```python
from build123d import *

# Parameters (mm, degrees)
F0_W             = 25.4
F0_H             = 25.4
F1_DEPTH         = 12.7
F3_D             = 3.175
F5_D             = 3.175
F7_D             = 3.175
F11_D            = 17.145
F11_DEPTH        = 3.81
F11_TIP          = 5.1508776566
F11_ON_F6_D      = 17.145
F11_ON_F6_DEPTH  = 3.81
F11_ON_F6_TIP    = 5.1508776566
F11_ON_F10_D     = 17.145
F11_ON_F10_DEPTH = 3.81
F11_ON_F10_TIP   = 5.1508776566
F11_ON_F4_D      = 17.145
F11_ON_F4_DEPTH  = 3.81
F11_ON_F4_TIP    = 5.1508776566
F11_ON_F9_D      = 17.145
F11_ON_F9_DEPTH  = 3.81
F11_ON_F9_TIP    = 5.1508776566
F11_ON_F2_D      = 17.145
F11_ON_F2_DEPTH  = 3.81
F11_ON_F2_TIP    = 5.1508776566
F12_D            = 22.225
F12_DEPTH        = 0.635
F12_TIP          = 6.6770636289
F12_ON_F2_D      = 22.225
F12_ON_F2_DEPTH  = 0.635
F12_ON_F2_TIP    = 6.6770636289
F12_ON_F10_D     = 22.225
F12_ON_F10_DEPTH = 0.635
F12_ON_F10_TIP   = 6.6770636289
F12_ON_F8_D      = 22.225
F12_ON_F8_DEPTH  = 0.635
F12_ON_F8_TIP    = 6.6770636289
F12_ON_F4_D      = 22.225
F12_ON_F4_DEPTH  = 0.635
F12_ON_F4_TIP    = 6.6770636289
F12_ON_F6_D      = 22.225
F12_ON_F6_DEPTH  = 0.635
F12_ON_F6_TIP    = 6.6770636289
F13_D            = 12.065
F13_DEPTH        = 3.81
F13_START        = 5.336186
F13_TIP          = 3.6246916843
F13_ON_F8_D      = 12.065
F13_ON_F8_DEPTH  = 3.81
F13_ON_F8_START  = 5.336186
F13_ON_F8_TIP    = 3.6246916843
F13_ON_F10_D     = 12.065
F13_ON_F10_DEPTH = 3.81
F13_ON_F10_START = 5.336186
F13_ON_F10_TIP   = 3.6246916843
F13_ON_F9_D      = 12.065
F13_ON_F9_DEPTH  = 3.81
F13_ON_F9_START  = 5.336186
F13_ON_F9_TIP    = 3.6246916843
F13_ON_F6_D      = 12.065
F13_ON_F6_DEPTH  = 3.81
F13_ON_F6_START  = 5.336186
F13_ON_F6_TIP    = 3.6246916843
F13_ON_F2_D      = 12.065
F13_ON_F2_DEPTH  = 3.81
F13_ON_F2_START  = 5.336186
F13_ON_F2_TIP    = 3.6246916843


with BuildPart() as f1:
    # F0 (on Top) → F1 (new body, symmetric)
    with BuildSketch(Plane.XY):
        Rectangle(F0_W, F0_H)
    extrude(amount=F1_DEPTH, both=True)

    # F3 (through all)
    with Locations(Plane.XY.offset(12.7)):
        with Locations((0, 0)):
            Hole(F3_D / 2)

    # F5 (through all)
    with Locations(Plane(origin=(-12.7, 0, 0), x_dir=(0, -1, 0), z_dir=(-1, 0, 0))):
        with Locations((0, 0)):
            Hole(F5_D / 2)

    # F7 (through all)
    with Locations(Plane(origin=(0, 12.7, 0), x_dir=(-1, 0, 0), z_dir=(0, 1, 0))):
        with Locations((0, 0)):
            Hole(F7_D / 2)

    # F11
    with Locations(Plane(origin=(0, 0, -12.7), x_dir=(1, 0, 0), z_dir=(0, 0, -1))):
        with Locations((0, 0)):
            Hole(F11_D / 2, depth=F11_DEPTH)
            with Locations((0, 0, -(F11_DEPTH + F11_TIP / 2))):  # 118° drill point
                Cone(0, F11_D / 2, F11_TIP, mode=Mode.SUBTRACT)

    # F11 on F6
    with Locations(Plane(origin=(0, 12.7, 0), x_dir=(-1, 0, 0), z_dir=(0, 1, 0))):
        with Locations((0, 0)):
            Hole(F11_ON_F6_D / 2, depth=F11_ON_F6_DEPTH)
            with Locations((0, 0, -(F11_ON_F6_DEPTH + F11_ON_F6_TIP / 2))):  # 118° drill point
                Cone(0, F11_ON_F6_D / 2, F11_ON_F6_TIP, mode=Mode.SUBTRACT)

    # F11 on F10
    with Locations(Plane.XZ.offset(12.7)):
        with Locations((0, 0)):
            Hole(F11_ON_F10_D / 2, depth=F11_ON_F10_DEPTH)
            with Locations((0, 0, -(F11_ON_F10_DEPTH + F11_ON_F10_TIP / 2))):  # 118° drill point
                Cone(0, F11_ON_F10_D / 2, F11_ON_F10_TIP, mode=Mode.SUBTRACT)

    # F11 on F4
    with Locations(Plane(origin=(-12.7, 0, 0), x_dir=(0, -1, 0), z_dir=(-1, 0, 0))):
        with Locations((0, 0)):
            Hole(F11_ON_F4_D / 2, depth=F11_ON_F4_DEPTH)
            with Locations((0, 0, -(F11_ON_F4_DEPTH + F11_ON_F4_TIP / 2))):  # 118° drill point
                Cone(0, F11_ON_F4_D / 2, F11_ON_F4_TIP, mode=Mode.SUBTRACT)

    # F11 on F9
    with Locations(Plane.YZ.offset(12.7)):
        with Locations((0, 0)):
            Hole(F11_ON_F9_D / 2, depth=F11_ON_F9_DEPTH)
            with Locations((0, 0, -(F11_ON_F9_DEPTH + F11_ON_F9_TIP / 2))):  # 118° drill point
                Cone(0, F11_ON_F9_D / 2, F11_ON_F9_TIP, mode=Mode.SUBTRACT)

    # F11 on F2
    with Locations(Plane.XY.offset(12.7)):
        with Locations((0, 0)):
            Hole(F11_ON_F2_D / 2, depth=F11_ON_F2_DEPTH)
            with Locations((0, 0, -(F11_ON_F2_DEPTH + F11_ON_F2_TIP / 2))):  # 118° drill point
                Cone(0, F11_ON_F2_D / 2, F11_ON_F2_TIP, mode=Mode.SUBTRACT)

    # F12
    with Locations(Plane.YZ.offset(12.7)):
        with Locations((0, 0)):
            Hole(F12_D / 2, depth=F12_DEPTH)
            with Locations((0, 0, -(F12_DEPTH + F12_TIP / 2))):  # 118° drill point
                Cone(0, F12_D / 2, F12_TIP, mode=Mode.SUBTRACT)

    # F12 on F2
    with Locations(Plane.XY.offset(12.7)):
        with Locations((0, 0)):
            Hole(F12_ON_F2_D / 2, depth=F12_ON_F2_DEPTH)
            with Locations((0, 0, -(F12_ON_F2_DEPTH + F12_ON_F2_TIP / 2))):  # 118° drill point
                Cone(0, F12_ON_F2_D / 2, F12_ON_F2_TIP, mode=Mode.SUBTRACT)

    # F12 on F10
    with Locations(Plane.XZ.offset(12.7)):
        with Locations((0, 0)):
            Hole(F12_ON_F10_D / 2, depth=F12_ON_F10_DEPTH)
            with Locations((0, 0, -(F12_ON_F10_DEPTH + F12_ON_F10_TIP / 2))):  # 118° drill point
                Cone(0, F12_ON_F10_D / 2, F12_ON_F10_TIP, mode=Mode.SUBTRACT)

    # F12 on F8
    with Locations(Plane(origin=(0, 0, -12.7), x_dir=(1, 0, 0), z_dir=(0, 0, -1))):
        with Locations((0, 0)):
            Hole(F12_ON_F8_D / 2, depth=F12_ON_F8_DEPTH)
            with Locations((0, 0, -(F12_ON_F8_DEPTH + F12_ON_F8_TIP / 2))):  # 118° drill point
                Cone(0, F12_ON_F8_D / 2, F12_ON_F8_TIP, mode=Mode.SUBTRACT)

    # F12 on F4
    with Locations(Plane(origin=(-12.7, 0, 0), x_dir=(0, -1, 0), z_dir=(-1, 0, 0))):
        with Locations((0, 0)):
            Hole(F12_ON_F4_D / 2, depth=F12_ON_F4_DEPTH)
            with Locations((0, 0, -(F12_ON_F4_DEPTH + F12_ON_F4_TIP / 2))):  # 118° drill point
                Cone(0, F12_ON_F4_D / 2, F12_ON_F4_TIP, mode=Mode.SUBTRACT)

    # F12 on F6
    with Locations(Plane(origin=(0, 12.7, 0), x_dir=(-1, 0, 0), z_dir=(0, 1, 0))):
        with Locations((0, 0)):
            Hole(F12_ON_F6_D / 2, depth=F12_ON_F6_DEPTH)
            with Locations((0, 0, -(F12_ON_F6_DEPTH + F12_ON_F6_TIP / 2))):  # 118° drill point
                Cone(0, F12_ON_F6_D / 2, F12_ON_F6_TIP, mode=Mode.SUBTRACT)

    # F13
    # its depths count from where the whole tool has entered the part; down to there all is cleared
    with Locations(Plane(origin=(-12.7, 0, 0), x_dir=(0, -1, 0), z_dir=(-1, 0, 0))):
        with Locations((0, 0)):
            Hole(F13_D / 2, depth=F13_START)
    with Locations(Plane(origin=(-12.7, 0, 0), x_dir=(0, -1, 0), z_dir=(-1, 0, 0)).offset(-F13_START)):
        with Locations((0, 0)):
            Hole(F13_D / 2, depth=F13_DEPTH)
            with Locations((0, 0, -(F13_DEPTH + F13_TIP / 2))):  # 118° drill point
                Cone(0, F13_D / 2, F13_TIP, mode=Mode.SUBTRACT)

    # F13 on F8
    # its depths count from where the whole tool has entered the part; down to there all is cleared
    with Locations(Plane(origin=(0, 0, -12.7), x_dir=(1, 0, 0), z_dir=(0, 0, -1))):
        with Locations((0, 0)):
            Hole(F13_ON_F8_D / 2, depth=F13_ON_F8_START)
    with Locations(Plane(origin=(0, 0, -12.7), x_dir=(1, 0, 0), z_dir=(0, 0, -1)).offset(-F13_ON_F8_START)):
        with Locations((0, 0)):
            Hole(F13_ON_F8_D / 2, depth=F13_ON_F8_DEPTH)
            with Locations((0, 0, -(F13_ON_F8_DEPTH + F13_ON_F8_TIP / 2))):  # 118° drill point
                Cone(0, F13_ON_F8_D / 2, F13_ON_F8_TIP, mode=Mode.SUBTRACT)

    # F13 on F10
    # its depths count from where the whole tool has entered the part; down to there all is cleared
    with Locations(Plane.XZ.offset(12.7)):
        with Locations((0, 0)):
            Hole(F13_ON_F10_D / 2, depth=F13_ON_F10_START)
    with Locations(Plane.XZ.offset(12.7).offset(-F13_ON_F10_START)):
        with Locations((0, 0)):
            Hole(F13_ON_F10_D / 2, depth=F13_ON_F10_DEPTH)
            with Locations((0, 0, -(F13_ON_F10_DEPTH + F13_ON_F10_TIP / 2))):  # 118° drill point
                Cone(0, F13_ON_F10_D / 2, F13_ON_F10_TIP, mode=Mode.SUBTRACT)

    # F13 on F9
    # its depths count from where the whole tool has entered the part; down to there all is cleared
    with Locations(Plane.YZ.offset(12.7)):
        with Locations((0, 0)):
            Hole(F13_ON_F9_D / 2, depth=F13_ON_F9_START)
    with Locations(Plane.YZ.offset(12.7).offset(-F13_ON_F9_START)):
        with Locations((0, 0)):
            Hole(F13_ON_F9_D / 2, depth=F13_ON_F9_DEPTH)
            with Locations((0, 0, -(F13_ON_F9_DEPTH + F13_ON_F9_TIP / 2))):  # 118° drill point
                Cone(0, F13_ON_F9_D / 2, F13_ON_F9_TIP, mode=Mode.SUBTRACT)

    # F13 on F6
    # its depths count from where the whole tool has entered the part; down to there all is cleared
    with Locations(Plane(origin=(0, 12.7, 0), x_dir=(-1, 0, 0), z_dir=(0, 1, 0))):
        with Locations((0, 0)):
            Hole(F13_ON_F6_D / 2, depth=F13_ON_F6_START)
    with Locations(Plane(origin=(0, 12.7, 0), x_dir=(-1, 0, 0), z_dir=(0, 1, 0)).offset(-F13_ON_F6_START)):
        with Locations((0, 0)):
            Hole(F13_ON_F6_D / 2, depth=F13_ON_F6_DEPTH)
            with Locations((0, 0, -(F13_ON_F6_DEPTH + F13_ON_F6_TIP / 2))):  # 118° drill point
                Cone(0, F13_ON_F6_D / 2, F13_ON_F6_TIP, mode=Mode.SUBTRACT)

    # F13 on F2
    # its depths count from where the whole tool has entered the part; down to there all is cleared
    with Locations(Plane.XY.offset(12.7)):
        with Locations((0, 0)):
            Hole(F13_ON_F2_D / 2, depth=F13_ON_F2_START)
    with Locations(Plane.XY.offset(12.7).offset(-F13_ON_F2_START)):
        with Locations((0, 0)):
            Hole(F13_ON_F2_D / 2, depth=F13_ON_F2_DEPTH)
            with Locations((0, 0, -(F13_ON_F2_DEPTH + F13_ON_F2_TIP / 2))):  # 118° drill point
                Cone(0, F13_ON_F2_D / 2, F13_ON_F2_TIP, mode=Mode.SUBTRACT)


solid = f1.part
```
Geometry: final body of the model. Coordinates: model frame, mm. A direction names the side the tool comes from. Coordinates: 2 decimals unless noted, no trailing zeros. Write each question's results on one line, items separated by ' | '.
1) Pull-direction query (Z, two-part tool) for faces 4 (the cylindrical face through (-10.6, -3.34, -12.38)), 5 (the cylindrical face through (-9.703, 4.609, 7.228)), 6 (the cylindrical face through (6.482, 4.446, 4.077)), 7 (the conical face through (-1.342, 6.044, -7.459)); classes: pulls with the +Z half, pulls with the -Z half, needs draft (parallel to the pull), parting line crosses it, or undercut.
Results list:
face 4: needs draft | face 5: undercut | face 6: undercut | face 7: pulls with the -Z half
2) Line query: line 1 (X direction, y = -5.75, z = 3.5); line 2 (X direction, y = -4, z = -5); line 3 (Z direction, x = 12.4, y = 0). Output: solid intervals per line, ascending. Write a range as from..to.
Results list:
line 1: -7.78..-4.91, 4.91..7.78 | line 2: -7.59..-4.52, 4.52..7.59 | line 3: -12.7..-11.11, 11.11..12.7
3) Pin query (flat end, axial travel): pin 1 (5 mm diameter, centred on x = 3.5, z = 6.5, fed in from +Y); pin 2 (1.5 mm diameter, centred on x = -2.5, z = 6, fed in from -Y); pin 3 (1 mm diameter, centred on x = 5, z = -5.5, fed in from +Y). Return the tip coordinate at first contact, or that it passes through.
Results list:
pin 1: y = 11.33 | pin 2: y = -8.1 | pin 3: y = 8.51
4) Section A-A, the plane z = 0. State how many separate pieces and enclosed holes the cut face has, plus the area to 3 significant figures.
Results list:
separate pieces: 4 | enclosed holes: 0 | area: 56.5 mm^2
5) Set-up query: faces 1 (the cylindrical face through (-12.38, 10.6, 3.34)), 2 (the cylindrical face through (-4.609, -7.228, -9.703)), 3 (the cylindrical face through (9.7, -8.18, 2.57)). Return all of +Z, -Z, +X, -X, +Y, -Y with unobstructed straight access to the full face (end or side cutting, diameter ignored); none if empty.
Results list:
face 1: -X | face 2: -Z | face 3: +X
